from build123d import *

# Parameters (mm, degrees)
F0_W     = 5
F0_H     = 5
F0_W_2   = 10
F1_DEPTH = 15
F2_DEPTH = 5
F3_W     = 5
F3_H     = 5
F4_DEPTH = 5
F5_W     = 10
F5_H     = 5
F6_DEPTH = 5
F5_W_2   = 5
F7_DEPTH = 5


with BuildPart() as f1:
    # F0 (on Front) → F1 (new body)
    with BuildSketch(Plane.XZ):
        with Locations((2.5, 2.5)):
            Rectangle(F0_W, F0_H)
        with Locations((7.5, 2.5)):
            Rectangle(F0_W, F0_H)
        with Locations((2.5, 7.5)):
            Rectangle(F0_W, F0_H)
        with Locations((15, 2.5)):
            Rectangle(F0_W_2, F0_H)
    extrude(amount=F1_DEPTH)

    # F0 (on Front) → F2 (cut)
    with BuildSketch(Plane.XZ):
        with Locations((2.5, 7.5)):
            Rectangle(F0_W, F0_H)
    extrude(amount=F2_DEPTH, mode=Mode.SUBTRACT)

    # F3 (on face) → F4 (cut)
    with BuildSketch(Plane.YZ.offset(5)):
        with Locations((-12.5, 7.5)):
            Rectangle(F3_W, F3_H)
    extrude(amount=-F4_DEPTH, mode=Mode.SUBTRACT)

    # F5 (on face) → F6 (cut)
    with BuildSketch(Plane.XY.offset(5)):
        with Locations((15, -12.5)):
            Rectangle(F5_W, F5_H)
    extrude(amount=-F6_DEPTH, mode=Mode.SUBTRACT)

    # F5 (on face) → F7 (cut)
    with BuildSketch(Plane.XY.offset(5)):
        with Locations((17.5, -2.5)):
            Rectangle(F5_W_2, F5_H)
    extrude(amount=-F7_DEPTH, mode=Mode.SUBTRACT)


solid = f1.part
CAD build for the part. Positions are in the model's coordinates, mm. A direction names the side the tool comes from. Round coordinates to 2 decimals unless told otherwise and drop trailing zeros. Loops run counter-clockwise (first coordinate to the right, second up) from the corner with the lowest first, then second, coordinate; pieces in that order, holes last.
(1) Cut at C-C (x = 11.5). Give the cut face in (y, z), plus the area to 3 significant figures.
(2) Cut at B-B (y = -9.25). Give the cut face in (x, z).
(3) Cut at A-A (z = 2.75). Give the cut face in (x, y), plus the area to 3 significant figures.
(4) Wall check: line 1 along X through (y, z) = (-8.75, 5.5); line 2 along Y through (x, z) = (2, 8.5). Give the ranges that are in metal, low to high.
(5) Which spindle directions (+Z, -Z, +X, -X, +Y, -Y) get a long thin tool onto all of the face, cutting with end or side? Do faces 1 (the flat face through (5, -7, 7)), 2 (the flat face through (15, -3, 3)), 3 (the flat face through (15, -10, 3)), 4 (the flat face through (3, -10, 7)), 5 (the flat face through (2, -5, 8)). Say none if no direction does.
(6) Drop flat-ended pins along their axis: pin 1 (1 mm diameter, centred on y = -5, z = 8, fed in from -X); pin 2 (3 mm diameter, centred on x = 11, y = -7.5, fed in from +Z); pin 3 (4 mm diameter, centred on y = -13, z = 2, fed in from +X); pin 4 (2.5 mm diameter, centred on y = -8.5, z = 8, fed in from +X). Give the stop position or say it passes through.
(7) Cut at D-D (x = 8.5). Give the cut face in (y, z).
Findings below:
1. outline: (-10, 0) - (0, 0) - (0, 5) - (-10, 5) - close
1. area: 50.0 mm2
2. outline: (0, 0) - (20, 0) - (20, 5) - (5, 5) - (5, 10) - (0, 10) - close
3. outline: (0, -15) - (10, -15) - (10, -10) - (20, -10) - (20, -5) - (15, -5) - (15, 0) - (0, 0) - close
3. area: 225 mm2
4. line 1: x = 0 to 5
4. line 2: y = -10 to -5
5. face 1: +Z, +X, +Y, -Y
5. face 2: +Z, -Z, +X, +Y
5. face 3: +Z, -Z, +X, -Y
5. face 4: +Z, +X, -X, -Y
5. face 5: +Z, +X, -X, +Y
6. pin 1: stops at x = 0
6. pin 2: stops at z = 5
6. pin 3: stops at x = 10
6. pin 4: stops at x = 5
7. outline: (-15, 0) - (0, 0) - (0, 5) - (-15, 5) - close
